from build123d import *

# Parameters (mm, degrees)
SCHIZZO1_R                   = 10
ESTRUSIONE_ESTRUSIONE1_DEPTH = 1000
SCHIZZO2_OUTSIDE_W           = 222.08
SCHIZZO2_OUTSIDE_H           = 222.08
SCHIZZO2_OUTSIDE_R           = 8.5
TAGLIO_ESTRUSIONE3_DEPTH     = 156
SCHIZZO3_OUTSIDE_W           = 222.08
SCHIZZO3_OUTSIDE_H           = 222.08
SCHIZZO3_OUTSIDE_R           = 8.5
TAGLIO_ESTRUSIONE4_DEPTH     = 50
SCHIZZO6_OUTSIDE_W           = 222.08
SCHIZZO6_OUTSIDE_H           = 222.08
SCHIZZO6_OUTSIDE_R           = 8
TAGLIO_ESTRUSIONE6_DEPTH     = 40
SCHIZZO7_W                   = 2.140478466
SCHIZZO7_H                   = 11.058829026
TAGLIO_ESTRUSIONE11_DEPTH    = 10


with BuildPart() as part:
    # Schizzo1 → Estrusione-Estrusione1 (new body)
    with BuildSketch(Plane.XY):
        Circle(SCHIZZO1_R)
    extrude(amount=ESTRUSIONE_ESTRUSIONE1_DEPTH)

    # Schizzo2 outside → Taglio-Estrusione3 (cut)
    with BuildSketch(Plane.XY.offset(1000)):
        Rectangle(SCHIZZO2_OUTSIDE_W, SCHIZZO2_OUTSIDE_H)
        Circle(SCHIZZO2_OUTSIDE_R, mode=Mode.SUBTRACT)
    extrude(amount=-TAGLIO_ESTRUSIONE3_DEPTH, mode=Mode.SUBTRACT)

    # Schizzo3 outside → Taglio-Estrusione4 (cut)
    with BuildSketch(Plane(origin=(0, 0, 0), x_dir=(-1, 0, 0), z_dir=(0, 0, -1))):
        Rectangle(SCHIZZO3_OUTSIDE_W, SCHIZZO3_OUTSIDE_H)
        Circle(SCHIZZO3_OUTSIDE_R, mode=Mode.SUBTRACT)
    extrude(amount=-TAGLIO_ESTRUSIONE4_DEPTH, mode=Mode.SUBTRACT)

    # Schizzo6 outside → Taglio-Estrusione6 (cut)
    with BuildSketch(Plane.XY.offset(1000)):
        Rectangle(SCHIZZO6_OUTSIDE_W, SCHIZZO6_OUTSIDE_H)
        Circle(SCHIZZO6_OUTSIDE_R, mode=Mode.SUBTRACT)
    extrude(amount=-TAGLIO_ESTRUSIONE6_DEPTH, mode=Mode.SUBTRACT)

    # Schizzo7 → Taglio-Estrusione11 (cut)
    with BuildSketch(Plane(origin=(0, 0, 0), x_dir=(-1, 0, 0), z_dir=(0, 0, -1))):
        with Locations((-1.070239233, 5.529414513)):
            Rectangle(SCHIZZO7_W, SCHIZZO7_H)
    extrude(amount=-TAGLIO_ESTRUSIONE11_DEPTH, mode=Mode.SUBTRACT)


solid = part.part
Can you work these out from the model? Positions are in its coordinate system, mm. A direction names the side the tool comes from. Coordinates: 2 decimals unless noted, no trailing zeros. Order: outer loops, then holes, each group sorted by start corner. A loop starts at its lowest first (then second) coordinate and runs counter-clockwise, first axis right, second up. Notation, with made-up numbers: (-6.5, 31) -> (27.5, 31) arc R32 cw to (27.5, 65) -> close; hole circle Ø1 at (60.25, 67.25). An arc over 180 degrees is marked (long way). Use one line per item in the form item = value.
Q1. Imagine slicing it at B-B, the plane z = 666. List the corners of the cut face in (x, y) for me.
From the geometry:
outline = circle Ø20 at (0, 0)
Q2. I need wall thicknesses on L1, parallel to X at y = -5, z = 729; L2, parallel to Y at x = 0.25, z = 645.5; L3, parallel to Z at x = 1.75, y = 6.5. Which ranges of each line are inside material? Lowest first, please.
From the geometry:
L1 = -8.66 to 8.66
L2 = -10 to 10
L3 = 10 to 1000
Q3. Imagine slicing it at A-A, the plane y = -3.75. List the corners of the cut face in (x, z) for me.
From the geometry:
outline = (-9.27, 50) -> (-7.63, 50) -> (-7.63, 0) -> (7.63, 0) -> (7.63, 50) -> (9.27, 50) -> (9.27, 844) -> (7.63, 844) -> (7.63, 960) -> (7.07, 960) -> (7.07, 1000) -> (-7.07, 1000) -> (-7.07, 960) -> (-7.63, 960) -> (-7.63, 844) -> (-9.27, 844) -> close
Q4. Which directions (+Z, -Z, +X, -X, +Y, -Y) give clear straight access to the entire face, cutting with the end or side of a thin tool? Please do faces 1 (the face through (-4.5, -7.4, 844)), 2 (the face through (4.5, -7.4, 50)), 3 (the face through (0, -2, 0)).
From the geometry:
face_1 = +Z
face_2 = -Z
face_3 = -Z, +X, -X, +Y, -Y
Q5. Will these pins go through, and if not, where does the flat tip stop? P1, Ø2, axis at y = 3.5, z = 136, coming from the -X side; P2, Ø1, axis at y = -5.5, z = 446.5, coming from the -X side; P3, Ø1.5, axis at x = -1.5, z = 873, coming from the -Y side.
From the geometry:
P1 = -9.68
P2 = -8.66
P3 = -8.47
